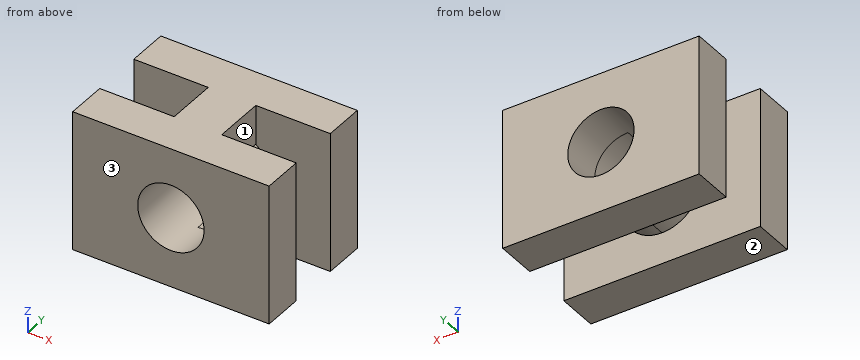
from build123d import *

# Parameters (mm, degrees)
BOSS_EXTRUDE1_DEPTH = 1.16
SKETCH2_W           = 8.88
SKETCH2_H           = 6.32
SKETCH2_R           = 1.5
BOSS_EXTRUDE2_DEPTH = 1.84


with BuildPart() as part:
    # Sketch1 → Boss-Extrude1 (new body)
    with BuildSketch(Plane(origin=(0, 0, 0), x_dir=(1, 0, 0), z_dir=(0, 1, 0))):
        with BuildLine():
            ThreePointArc((0, -1.75), (-0.568301, -1.655154), (-1.075, -1.380896))
            Line((-1.075, -1.380896), (-1.075, -3.16))
            Line((-1.075, -3.16), (0, -3.16))
            Line((0, -3.16), (0, -1.75))
        make_face()
        with BuildLine():
            ThreePointArc((1.075, -1.380896), (0.568301, -1.655154), (0, -1.75))
            Line((0, -1.75), (0, -3.16))
            Line((0, -3.16), (1.075, -3.16))
            Line((1.075, -3.16), (1.075, -1.380896))
        make_face()
        with BuildLine():
            ThreePointArc((0, 1.75), (-1.655154, 0.568301), (-1.075, -1.380896))
            ThreePointArc((-1.075, -1.380896), (-0.568301, -1.655154), (0, -1.75))
            Line((0, -1.75), (0, -1.5))
            ThreePointArc((0, -1.5), (-1.5, 0), (0, 1.5))
            Line((0, 1.5), (0, 1.75))
        make_face()
        with BuildLine():
            ThreePointArc((1.75, 0), (1.237437, 1.237437), (0, 1.75))
            Line((0, 1.75), (0, 1.5))
            ThreePointArc((0, 1.5), (1.06066, 1.06066), (1.5, 0))
            ThreePointArc((1.5, 0), (1.06066, -1.06066), (0, -1.5))
            Line((0, -1.5), (0, -1.75))
            ThreePointArc((0, -1.75), (0.568301, -1.655154), (1.075, -1.380896))
            ThreePointArc((1.075, -1.380896), (1.57222, -0.768521), (1.75, 0))
        make_face()
    boss_extrude1 = extrude(amount=BOSS_EXTRUDE1_DEPTH)

    # Sketch2 → Boss-Extrude2 (add)
    with BuildSketch(Plane(origin=(0, 1.16, 0), x_dir=(1, 0, 0), z_dir=(0, 1, 0))):
        Rectangle(SKETCH2_W, SKETCH2_H)
        with Locations(Location((0, 0, 0), (0, 0, 270))):
            Circle(SKETCH2_R, mode=Mode.SUBTRACT)
    boss_extrude2 = extrude(amount=BOSS_EXTRUDE2_DEPTH)

    # Mirror1: Boss-Extrude1, Boss-Extrude2 across plane
    add(boss_extrude1.mirror(Plane.ZX))
    add(boss_extrude2.mirror(Plane.ZX))


solid = part.part
Work out the finished part from the listing and answer in its coordinate system (mm). Face numbers are marked on the shaded views. Give positions to 0.01 mm unless a question says otherwise; leave off trailing zeros. Write each loop counter-clockwise with the first axis right and the second up, starting at its lowest first coordinate (ties: lowest second). Pieces come first, ordered by that corner, then holes. Notation, with made-up numbers: M -35,14.25 L -15,14.25 A31 ccw -15,45.25 Z; hole C 18,64 d6. An arc over 180 degrees is marked long. Answer as CSV lines item,"result".
Q1. A cutting plane is placed at C-C on y = -0.25. Write down the section's boundary in (x, z) (3 decimals).
A:
outline,"M -1.075,1.381 A1.75 ccw long 1.75,0 A1.75 ccw 1.075,1.381 L 1.075,3.16 L -1.075,3.16 Z; hole M 0,-1.5 A1.5 ccw 1.5,0 A1.5 ccw long Z"
Q2. A cutting plane is placed at D-D on z = 2.75. Write down the section's boundary in (x, y) (3 decimals).
A:
outline,"M -4.44,-3 L 4.44,-3 L 4.44,-1.16 L 1.075,-1.16 L 1.075,1.16 L 4.44,1.16 L 4.44,3 L -4.44,3 L -4.44,1.16 L -1.075,1.16 L -1.075,-1.16 L -4.44,-1.16 Z"
Q3. Find the intervals of material crossed by probe 1 along Y at (x, z) = (-2.75, 0); probe 2 along Z at (x, y) = (1.25, 0.2); probe 3 along Z at (x, y) = (1.25, 1.2), in increasing order. Write a range as [from, to].
A:
probe 1,"y = [-3, -1.16], [1.16, 3]"
probe 2,"z = [-1.22, -0.83], [0.83, 1.22]"
probe 3,"z = [-3.16, -0.83], [0.83, 3.16]"
Q4. A cutting plane is placed at B-B on z = -2.25. Write down the section's boundary in (x, y).
A:
outline,"M -4.44,-3 L 4.44,-3 L 4.44,-1.16 L -4.44,-1.16 Z; M -4.44,1.16 L 4.44,1.16 L 4.44,3 L -4.44,3 Z"
Q5. Given P1, Ø0.5, axis at y = 0, z = 2.5, coming from the +X side (3 decimals); P2, Ø0.5, axis at y = 0, z = 2, coming from the -X side (3 decimals), each flat-ended and moving along its own axis, determine where each tip first touches the part or whether it passes through.
A:
P1,"stops at x = 1.075"
P2,"stops at x = -1.075"
Q6. A cutting plane is placed at A-A on x = -3. Write down the section's boundary in (y, z), plus the area to 3 significant figures.
A:
outline,"M -3,-3.16 L -1.16,-3.16 L -1.16,3.16 L -3,3.16 Z; M 1.16,-3.16 L 3,-3.16 L 3,3.16 L 1.16,3.16 Z"
area,"23.3 mm²"
Q7. The mould has two halves that part along Y. Classify the marked faces 1, 2 and 3: +Y half, -Y half, draft (parallel to the pull), parting line (faces both ways), or undercut.
A:
face 1,"undercut"
face 2,"draft"
face 3,"-Y half"
